```python
from build123d import *

# Parameters (mm, degrees)
F0_R     = 23.20358
F1_DEPTH = 152.4


with BuildPart() as f1:
    # F0 (on Front) → F1 (new body)
    with BuildSketch(Plane.XZ):
        Circle(F0_R)
        with BuildLine():
            ThreePointArc((-2.96408, -17.995849), (-13.904967, -11.802045), (-18.238321, 0))
            Line((-18.238321, 0), (-2.96408, 0))
            Line((-2.96408, 0), (-2.96408, -17.995849))
        make_face(mode=Mode.SUBTRACT)
        with BuildLine():
            ThreePointArc((18.238321, 0), (12.89644, -12.89644), (0, -18.238321))
            Line((0, -18.238321), (0, 0))
            Line((0, 0), (18.238321, 0))
        make_face(mode=Mode.SUBTRACT)
        with BuildLine():
            ThreePointArc((-18.145688, 1.835854), (-13.292552, 12.487771), (-2.96408, 17.995849))
            Line((-2.96408, 17.995849), (-2.96408, 1.835854))
            Line((-2.96408, 1.835854), (-18.145688, 1.835854))
        make_face(mode=Mode.SUBTRACT)
        with BuildLine():
            Line((0, 3.556), (0, 18.238321))
            ThreePointArc((0, 18.238321), (12.289425, 13.476141), (18.161105, 1.676494))
            Line((18.161105, 1.676494), (0, 1.676494))
            Line((0, 1.676494), (0, 3.556))
        make_face(mode=Mode.SUBTRACT)
    extrude(amount=F1_DEPTH)


solid = f1.part
```
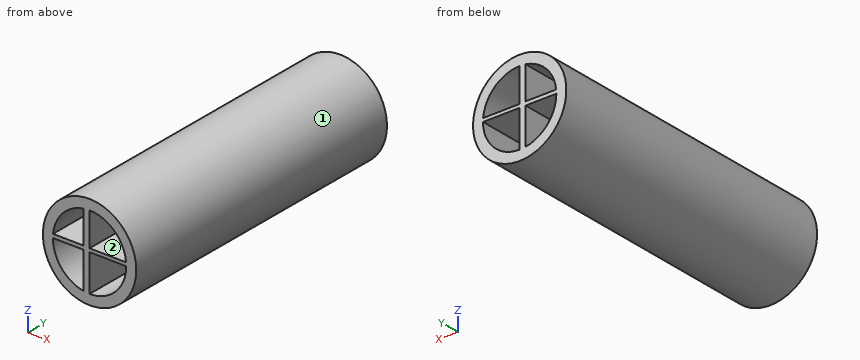
Here's how the part is built. I have some questions about the finished solid (model axes, mm). Face numbers are marked on the shaded views. Round coordinates to 2 decimals unless told otherwise and drop trailing zeros. Order: outer loops, then holes, each group sorted by start corner. A loop starts at its lowest first (then second) coordinate and runs counter-clockwise, first axis right, second up. Notation, with made-up numbers: M 55,28 L 100,28 A16 ccw 100,49 Z; hole C -25.75,-34.75 d3. An arc over 180 degrees is marked long. Use CSV: the item, a comma, the result in double quotes.
1) I'm going to push flat-ended pins straight in: P1, Ø4.5, axis at x = -8, y = -44, coming from the -Z side; P2, Ø4.5, axis at x = -12.5, y = -87, coming from the +Z side; P3, Ø8, axis at x = -13.5, y = -79.5, coming from the -Z side. Where does each tip first touch, or does it pass through?
Taken from the geometry:
P1,"z = -22.48"
P2,"z = 20.82"
P3,"z = -21.17"
2) I want a section at B-B (z = -10). List the corners of the cut face in (x, y) for me, then the cut area to 3 significant figures.
Taken from the geometry:
outline,"M -20.94,-152.4 L -15.25,-152.4 L -15.25,0 L -20.94,0 Z; M -2.96,-152.4 L 0,-152.4 L 0,0 L -2.96,0 Z; M 15.25,-152.4 L 20.94,-152.4 L 20.94,0 L 15.25,0 Z"
area,"2,180 mm^2"
3) I want a section at A-A (y = -90). List the corners of the cut face in (x, z) for me.
Taken from the geometry:
outline,"C 0,0 d46.41; hole M -18.24,0 A18.24 ccw -2.96,-18 L -2.96,0 Z; hole M -18.15,1.84 L -2.96,1.84 L -2.96,18 A18.24 ccw Z; hole M 0,-18.24 A18.24 ccw 18.24,0 L 0,0 Z; hole M 0,1.68 L 18.16,1.68 A18.24 ccw 0,18.24 Z"
4) I want a section at C-C (x = 11). List the corners of the cut face in (y, z) for me.
Taken from the geometry:
outline,"M -152.4,-20.43 L 0,-20.43 L 0,-14.55 L -152.4,-14.55 Z; M -152.4,0 L 0,0 L 0,1.68 L -152.4,1.68 Z; M -152.4,14.55 L 0,14.55 L 0,20.43 L -152.4,20.43 Z"
5) If we mould it in two halves opening along Z, with no side actions, what happens to the marked faces 1 and 2? For each: pulls with the +Z half, pulls with the -Z half, needs draft (parallel to the pull), parting line crosses it, or undercut.
Taken from the geometry:
face 1,"parting line crosses it"
face 2,"undercut"
6) I need wall thicknesses on line 1 along X through (y, z) = (-24.5, -9.5); line 2 along X through (y, z) = (-123, 16.5); line 3 along Z through (x, y) = (-12, -29). Which ranges of each line are inside material? Lowest first, please. Write a range as [from, to].
Taken from the geometry:
line 1,"[-21.17, -15.57], [-2.96, 0], [15.57, 21.17]"
line 2,"[-16.31, -7.77], [-2.96, 0], [7.77, 16.31]"
line 3,"[-19.86, -13.73], [0, 1.84], [13.73, 19.86]"
